Source: three-view drawing plus pictorial views. Frame: mm from the lowest corner of the part. Coordinates: 2 decimals unless noted, no trailing zeros. Order: outer loops, then holes, each group sorted by start corner. A loop starts at its lowest first (then second) coordinate and runs counter-clockwise, first axis right, second up. Notation, with made-up numbers: (62, 71) - (108, 71) arc R17 cw to (108, 85) - close; hole circle Ø8 at (19, 27). An arc over 180 degrees is marked (long way). Use a Markdown table: item, result. Add a question column.
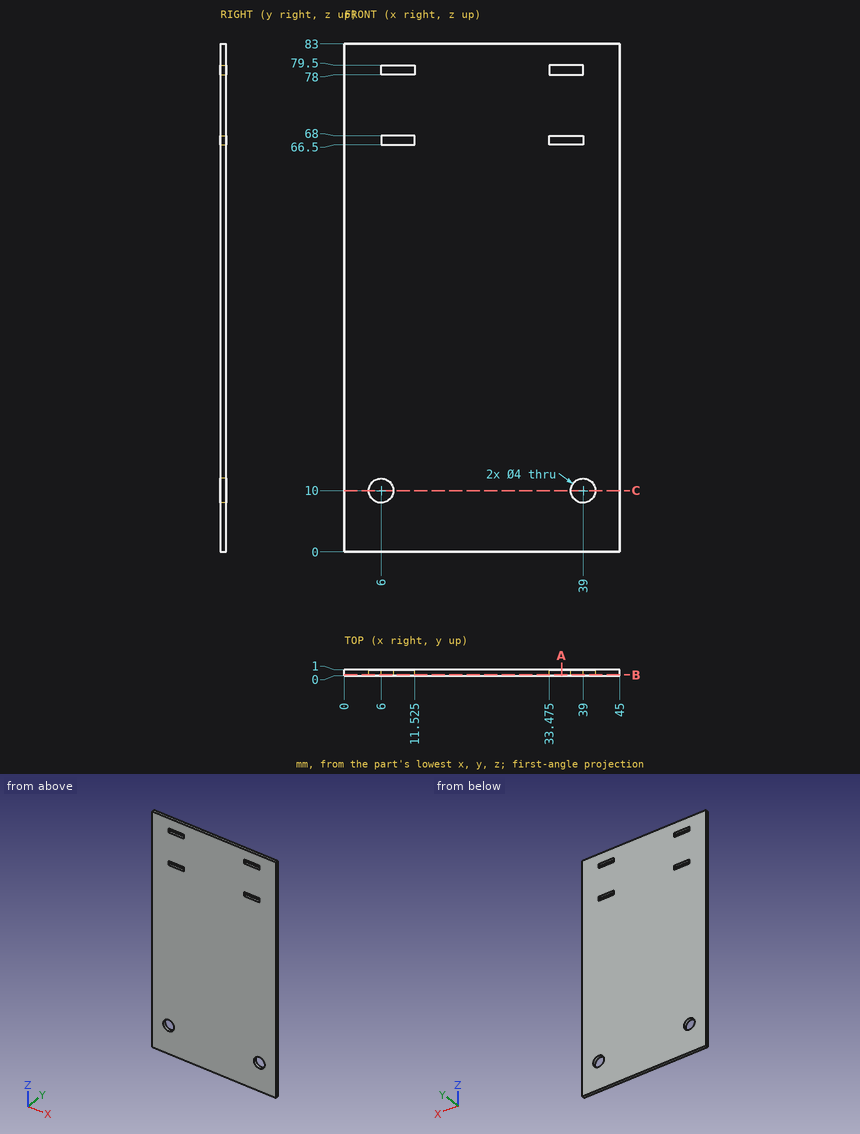
1) Pin query (flat end, axial travel): pin 1 (2.5 mm diameter, centred on x = 6, z = 10, fed in from -Y). Return the tip coordinate at first contact, or that it passes through.
2) Section A-A (x = 35.5). Return loops of the section in (y, z).
3) Section C-C (z = 10). Return loops of the section in (x, y), then the cut area to 3 significant figures.
4) Ray query, line 1 along Z through (x, y) = (10.5, 0.9); line 2 along X through (y, z) = (0.35, 79) (3 decimals). Return the intervals inside material, ascending.
5) Section B-B (y = 0.2). Return loops of the section in (x, z) (3 decimals), then the cut area to 3 significant figures.
Values follow:
| question | item | result |
|---|---|---|
| 1 | pin 1 | passes through |
| 2 | outline | (0, 0) - (1, 0) - (1, 66.5) - (0, 66.5) - close; (0, 68) - (1, 68) - (1, 78) - (0, 78) - close; (0, 79.5) - (1, 79.5) - (1, 83) - (0, 83) - close |
| 3 | outline | (0, 0) - (4, 0) - (4, 1) - (0, 1) - close; (8, 0) - (37, 0) - (37, 1) - (8, 1) - close; (41, 0) - (45, 0) - (45, 1) - (41, 1) - close |
| 3 | area | 37.0 mm² |
| 4 | line 1 | z = 0 to 66.5, 68 to 78, 79.5 to 83 |
| 4 | line 2 | x = 0 to 6, 11.525 to 33.475, 39 to 45 |
| 5 | outline | (0, 0) - (45, 0) - (45, 83) - (0, 83) - close; hole circle Ø4 at (6, 10); hole (6, 66.5) - (11.525, 66.5) - (11.525, 68) - (6, 68) - close; hole (6, 78) - (11.525, 78) - (11.525, 79.5) - (6, 79.5) - close; hole (33.475, 66.5) - (39, 66.5) - (39, 68) - (33.475, 68) - close; hole (33.475, 78) - (39, 78) - (39, 79.5) - (33.475, 79.5) - close; hole circle Ø4 at (39, 10) |
| 5 | area | 3,680 mm² |
